The figure shows three views and two pictorial views of one solid part (mm, origin at its lowest corner). Answer the questions. Give positions to 0.01 mm unless a question says otherwise; leave off trailing zeros. Loops run counter-clockwise (first coordinate to the right, second up) from the corner with the lowest first, then second, coordinate; pieces in that order, holes last. Notation, with made-up numbers: M -23.5,-7 L 24.5,-7 A14 cw 24.5,15 Z; hole C -39.5,79.25 d9. An arc over 180 degrees is marked long. Answer as a JSON object with one key per item and string values. Group by question number.
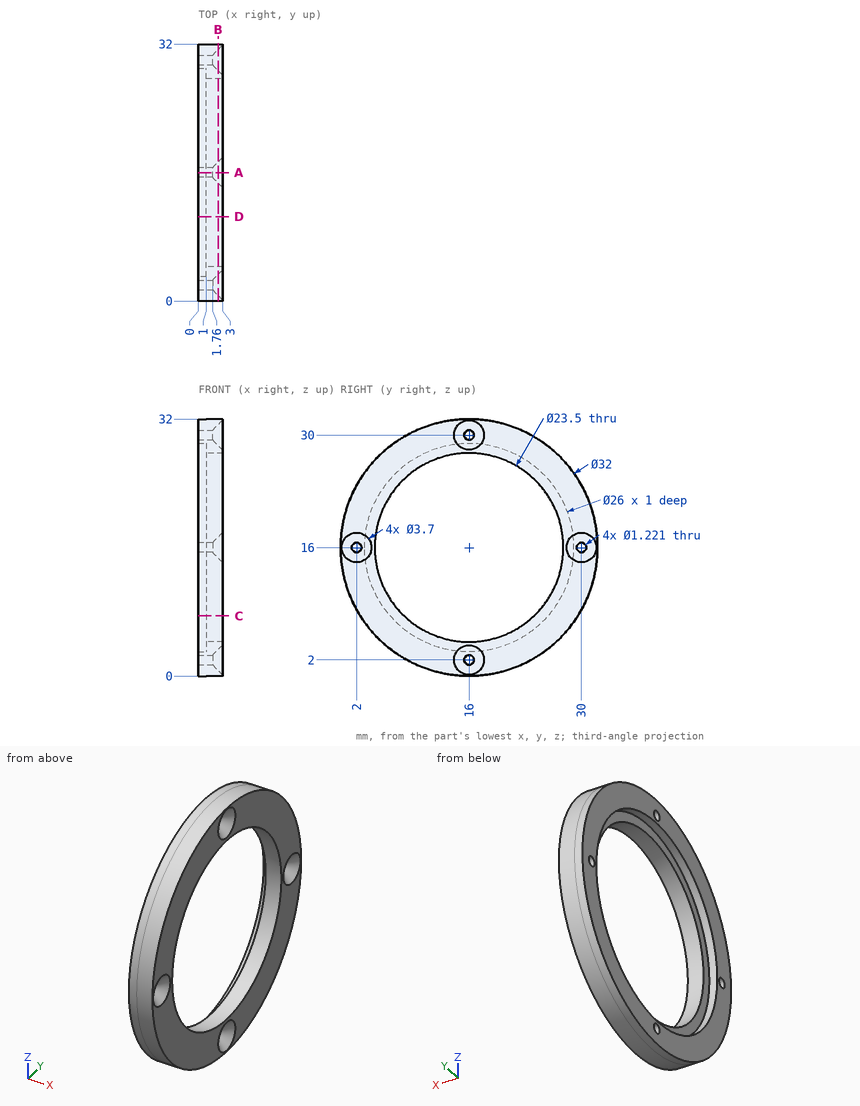
Item 1: Find the intervals of material crossed by probe 1 along Z at (x, y) = (0.45, 16); probe 2 along Z at (x, y) = (1.2, 16); probe 3 along Y at (x, z) = (2, 15.5) (1 decimal), in increasing order. Write a range as [from, to].
Item 2: A cutting plane is placed at B-B (x = 2.45). Determine the outline of the cut face in (y, z).
Item 3: A cutting plane is placed at C-C (z = 7.5). Determine the outline of the cut face in (x, y) (1 decimal).
Item 4: A cutting plane is placed at D-D (y = 10.5). Determine the outline of the cut face in (x, z) (1 decimal).
Item 5: Given pin 1 Ø1.4 at (y, z) = (30, 16) entering from +X; pin 2 Ø0.7 at (y, z) = (16, 30) entering from +X; pin 3 Ø3 at (y, z) = (14, 4.5) entering from +X, each flat-ended and moving along its own axis, determine where each tip first touches the part or whether it passes through.
Item 6: A cutting plane is placed at A-A (y = 16). Determine the outline of the cut face in (x, z).
The answers:
{
 "1": {"probe 1": "z = [0, 1.39], [2.61, 3], [29, 29.39], [30.61, 32]", "probe 2": "z = [0, 1.39], [2.61, 4.25], [27.75, 29.39], [30.61, 32]", "probe 3": "y = [0, 1.3], [2.7, 4.3], [27.7, 29.3], [30.7, 32]"},
 "2": {"outline": "C 16,16 d32; hole C 2,16 d2.6; hole C 16,16 d23.5; hole C 16,2 d2.6; hole C 16,30 d2.6; hole C 30,16 d2.6"},
 "3": {"outline": "M 0,2.4 L 3,2.4 L 3,7.9 L 1,7.9 L 1,6.2 L 0,6.2 Z; M 0,25.8 L 1,25.8 L 1,24.1 L 3,24.1 L 3,29.6 L 0,29.6 Z"},
 "4": {"outline": "M 0,1 L 3,1 L 3,5.6 L 1,5.6 L 1,4.2 L 0,4.2 Z; M 0,27.8 L 1,27.8 L 1,26.4 L 3,26.4 L 3,31 L 0,31 Z"},
 "5": {"pin 1": "stops at x = 1.85", "pin 2": "passes through", "pin 3": "stops at x = 3"},
 "6": {"outline": "M 0,0 L 3,0 L 3,0.15 L 1.76,1.39 L 0,1.39 Z; M 0,2.61 L 1.76,2.61 L 3,3.85 L 3,4.25 L 1,4.25 L 1,3 L 0,3 Z; M 0,29 L 1,29 L 1,27.75 L 3,27.75 L 3,28.15 L 1.76,29.39 L 0,29.39 Z; M 0,30.61 L 1.76,30.61 L 3,31.85 L 3,32 L 0,32 Z"}
}
